Part print with two shaded views. Sizes in mm from the minimum x, y, z corner. A direction names the side the tool comes from. Round coordinates to 2 decimals unless told otherwise and drop trailing zeros. Loops run counter-clockwise (first coordinate to the right, second up) from the corner with the lowest first, then second, coordinate; pieces in that order, holes last. Notation, with made-up numbers: (52, 32) - (86, 32) arc R19 ccw to (86, 60) - close; hole circle Ø10 at (76, 9). An arc over 180 degrees is marked (long way). Write each question's results on one line, items separated by ' | '. Start each with the question number.
(1) Cut at B-B, the plane y = 16. List the corners of the cut face in (x, z) (1 decimal).
(2) Tool access for the marked faces 1 and 2: list every direction of +Z, -Z, +X, -X, +Y, -Y with a clear straight run to the whole face (end or side of a thin tool).
(3) Drill centre lines: L1, parallel to Z at x = 1.25, y = 13.25; L2, parallel to Y at x = 15.25, z = 7.5 (1 decimal); L3, parallel to X at y = 15, z = 12.5 (1 decimal). Where is each one in solid material? Low to high.
(4) Flat gauge pins, fed straight in: P1, Ø10, axis at y = 6.5, z = 7, coming from the +X side; P2, Ø1, axis at x = 18.5, y = 4.5, coming from the -Z side; P3, Ø1, axis at x = 17.5, z = 5, coming from the -Y side; P4, Ø8, axis at x = 10.32, y = 10.32, coming from the -Z side. Where does each tip first touch, or does it go through?
(5) Cut at A-A, the plane z = 18.75. List the corners of the cut face in (x, y).
(6) Cut at D-D, the plane z = 13. List the corners of the cut face in (x, y), then the cut area to 3 significant figures.
(7) Mould opens along X. For the marked faces 3, 4 and 5 say: released by +X, released by -X, zero draft, split by the parting line, or undercut.
(8) Cut at C-C, the plane x = 12.5. List the corners of the cut face in (y, z) (1 decimal), then the cut area to 3 significant figures.
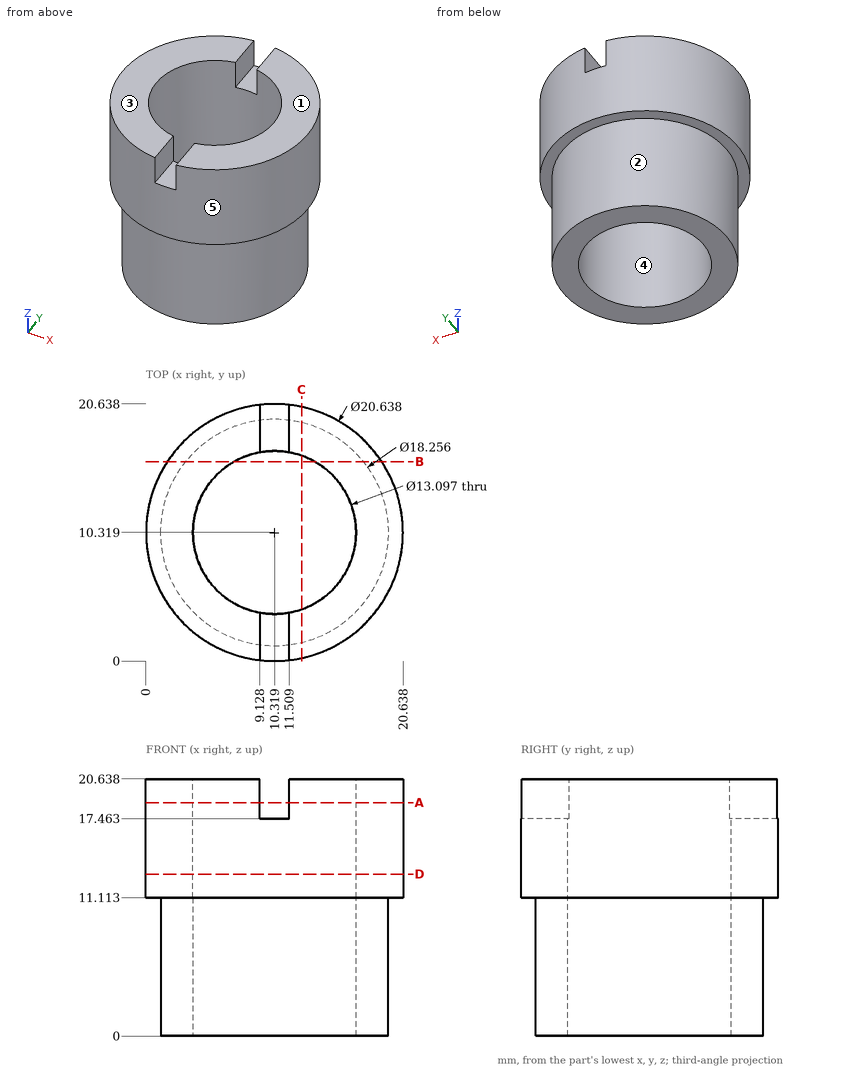
A:
1) outline: (1.7, 11.1) - (3.2, 11.1) - (3.2, 0) - (7.1, 0) - (7.1, 20.6) - (1.7, 20.6) - close; (13.6, 0) - (17.5, 0) - (17.5, 11.1) - (18.9, 11.1) - (18.9, 20.6) - (13.6, 20.6) - close
2) face 1: +Z, +X, -X, +Y, -Y | face 2: -Z
3) L1: 11.11 to 20.64 | L2: 2.6 to 6, 14.6 to 18 | L3: 1.1 to 5.7, 14.9 to 19.5
4) P1: x = 20.59 | P2: z = 11.11 | P3: y = 4.1 | P4: through
5) outline: (9.13, 0.07) - (9.13, 3.88) arc R6.55 cw to (9.13, 16.76) - (9.13, 20.57) arc R10.32 ccw to start; (11.51, 0.07) arc R10.32 ccw to (11.51, 20.57) - (11.51, 16.76) arc R6.55 cw to (11.51, 3.88) - close
6) outline: circle Ø20.64 at (10.32, 10.32); hole circle Ø13.1 at (10.32, 10.32) | area: 200 mm2
7) face 3: zero draft | face 4: undercut | face 5: split by the parting line
8) outline: (0.2, 11.1) - (1.5, 11.1) - (1.5, 0) - (4.1, 0) - (4.1, 20.6) - (0.2, 20.6) - close; (16.5, 0) - (19.2, 0) - (19.2, 11.1) - (20.4, 11.1) - (20.4, 20.6) - (16.5, 20.6) - close | area: 134 mm2
